Here's how the part is built. I have some questions about the finished solid (model axes, mm). A direction names the side the tool comes from. Give positions to 0.01 mm unless a question says otherwise; leave off trailing zeros. Loops run counter-clockwise (first coordinate to the right, second up) from the corner with the lowest first, then second, coordinate; pieces in that order, holes last. Notation, with made-up numbers: (46.5, 63) - (71.5, 63) arc R29 ccw to (71.5, 87) - close; hole circle Ø4 at (82, 62). An arc over 180 degrees is marked (long way). Use one line per item in the form item = value.
from build123d import *

# Parameters (mm, degrees)
SKETCH1_R           = 2
BOSS_EXTRUDE1_DEPTH = 5.5
CUT_EXTRUDE1_START  = -2.5
SKETCH2_R           = 3.5
SKETCH2_R_2         = 2
CUT_EXTRUDE1_DEPTH  = 2.5


with BuildPart() as part:
    # Sketch1 → Boss-Extrude1 (new body)
    with BuildSketch(Plane(origin=(0, 0, 0), x_dir=(1, 0, 0), z_dir=(0, 1, 0))):
        with BuildLine():
            Line((-4.5, 45.334635496), (-4.5, -45.334635496))
            ThreePointArc((-4.5, -45.334635496), (-4.998538124, -48.452683318), (-6.444444444, -51.259837998))
            ThreePointArc((-6.444444444, -51.259837998), (0, -64), (6.444444444, -51.259837998))
            ThreePointArc((6.444444444, -51.259837998), (4.998538124, -48.452683318), (4.5, -45.334635496))
            Line((4.5, -45.334635496), (4.5, 45.334635496))
            ThreePointArc((4.5, 45.334635496), (4.998538124, 48.452683318), (6.444444444, 51.259837998))
            ThreePointArc((6.444444444, 51.259837998), (0, 64), (-6.444444444, 51.259837998))
            ThreePointArc((-6.444444444, 51.259837998), (-4.998538124, 48.452683318), (-4.5, 45.334635496))
        make_face()
        with Locations(Location((0, 56, 0), (0, 0, 270))):
            Circle(SKETCH1_R, mode=Mode.SUBTRACT)
        with Locations(Location((0, -56, 0), (0, 0, 90))):
            Circle(SKETCH1_R, mode=Mode.SUBTRACT)
    extrude(amount=BOSS_EXTRUDE1_DEPTH)

    # Sketch2 → Cut-Extrude1 (cut)
    # profile 1 of 2: a face of its own
    with BuildSketch(Plane(origin=(0, 5.5, 0), x_dir=(1, 0, 0), z_dir=(0, 1, 0)).offset(CUT_EXTRUDE1_START)):
        with Locations(Location((0, 56, 0), (0, 0, 270))):
            Circle(SKETCH2_R)
        with Locations(Location((0, 56, 0), (0, 0, 270))):
            Circle(SKETCH2_R_2, mode=Mode.SUBTRACT)
    # profile 2 of 2: a face of its own
    with BuildSketch(Plane(origin=(0, 5.5, 0), x_dir=(1, 0, 0), z_dir=(0, 1, 0)).offset(CUT_EXTRUDE1_START)):
        with Locations(Location((0, -56, 0), (0, 0, 270))):
            Circle(SKETCH2_R)
        with Locations(Location((0, -56, 0), (0, 0, 90))):
            Circle(SKETCH2_R_2, mode=Mode.SUBTRACT)
    extrude(amount=CUT_EXTRUDE1_DEPTH, mode=Mode.SUBTRACT)


solid = part.part
(1) For P1, Ø5.5, axis at x = 0, z = 55.5, coming from the +Y side; P2, Ø2, axis at x = -5, y = 2, coming from the -Z side; P3, Ø1.5, axis at x = -6, y = 1.5, coming from the -Z side, each with a flat end and sliding along its axis, tell me the tip position at first contact or that it passes through.
Geometry says:
P1 = 3
P2 = -62.93
P3 = -62.04
(2) If we section it at B-B (z = -56): List the corners of the cut face in (x, y) for me.
Geometry says:
outline = (-8, 0) - (-2, 0) - (-2, 3) - (-3.5, 3) - (-3.5, 5.5) - (-8, 5.5) - close; (2, 0) - (8, 0) - (8, 5.5) - (3.5, 5.5) - (3.5, 3) - (2, 3) - close
(3) If we section it at A-A (y = 4): List the corners of the cut face in (x, z) for me, plus the area to 3 significant figures.
Geometry says:
outline = (-6.44, -51.26) arc R8 ccw (long way) to (6.44, -51.26) arc R10 cw to (4.5, -45.33) - (4.5, 45.33) arc R10 cw to (6.44, 51.26) arc R8 ccw (long way) to (-6.44, 51.26) arc R10 cw to (-4.5, 45.33) - (-4.5, -45.33) arc R10 cw to start; hole circle Ø7 at (0, -56); hole circle Ø7 at (0, 56)
area = 1,200 mm²
(4) For faces 1 (the cylindrical face through (4.985, 2.712, -48.41)), 2 (the cylindrical face through (-5.01, 2.71, -48.49)), 3 (the flat face through (0, 0, -1)), 4 (the flat face through (0, 5.5, -1)), 5 (the cylindrical face through (0.154, 4.232, -59.497)), which set-ups out of +Z, -Z, +X, -X, +Y, -Y let a thin tool reach every point of the face, with its end or its side?
Geometry says:
face_1 = +X, +Y, -Y
face_2 = -X, +Y, -Y
face_3 = +Z, -Z, +X, -X, -Y
face_4 = +Z, -Z, +X, -X, +Y
face_5 = +Y
(5) If we section it at C-C (x = 0): List the corners of the cut face in (y, z) for me, plus the area to 3 significant figures.
Geometry says:
outline = (0, -64) - (5.5, -64) - (5.5, -59.5) - (3, -59.5) - (3, -58) - (0, -58) - close; (0, -54) - (3, -54) - (3, -52.5) - (5.5, -52.5) - (5.5, 52.5) - (3, 52.5) - (3, 54) - (0, 54) - close; (0, 58) - (3, 58) - (3, 59.5) - (5.5, 59.5) - (5.5, 64) - (0, 64) - close
area = 645 mm²
(6) If I drill on probe 1 along Z at (x, y) = (0.25, 2.65); probe 2 along X at (y, z) = (1.5, 56); probe 3 along X at (y, z) = (3.9, 46), over which ranges is the centre line in solid material (lowest first)?
Geometry says:
probe_1 = -64 to -57.98, -54.02 to 54.02, 57.98 to 64
probe_2 = -8 to -2, 2 to 8
probe_3 = -4.52 to 4.52
